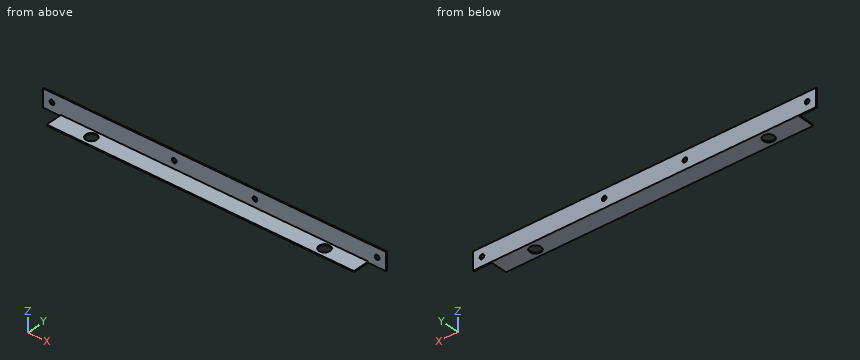
```python
from build123d import *

# Parameters (mm, degrees)
F1_DEPTH = 242.8875
F2_R     = 7.9375
F2_W     = 25.4
F2_H     = 23.8125
F4_DEPTH = 25.4
F3_R     = 3.302
F5_DEPTH = 25.4


with BuildPart() as f1:
    # F0 (on Right) → F1 (new body, symmetric)
    with BuildSketch(Plane.YZ):
        Polygon((0, 0), (0, 25.4), (-1.5875, 25.4), (-1.5875, 1.5875), (-25.4, 1.5875), (-25.4, 0), align=None)
    extrude(amount=F1_DEPTH, both=True)

    # F2 (on face) → F4 (cut)
    with BuildSketch(Plane(origin=(0, 0, 0), x_dir=(1, 0, 0), z_dir=(0, 0, -1))):
        with Locations((-165.1, 12.7)):
            Circle(F2_R)
        with Locations((165.1, 12.7)):
            Circle(F2_R)
        with Locations((-230.1875, 13.49375)):
            Rectangle(F2_W, F2_H)
        with Locations((230.1875, 13.49375)):
            Rectangle(F2_W, F2_H)
    extrude(amount=-F4_DEPTH, mode=Mode.SUBTRACT)

    # F3 (on face) → F5 (cut)
    with BuildSketch(Plane.XZ.offset(1.5875)):
        with Locations((-230.1875, 12.7)):
            Circle(F3_R)
        with Locations((230.1875, 12.7)):
            Circle(F3_R)
        with Locations((-57.15, 12.7)):
            Circle(F3_R)
        with Locations((57.15, 12.7)):
            Circle(F3_R)
    extrude(amount=-F5_DEPTH, mode=Mode.SUBTRACT)


solid = f1.part
```
Part model, mm, in its own coordinate system. Coordinates: 2 decimals unless noted, no trailing zeros. Order: outer loops, then holes, each group sorted by start corner. A loop starts at its lowest first (then second) coordinate and runs counter-clockwise, first axis right, second up. Notation, with made-up numbers: (64, 63) - (79, 63) arc R10 ccw to (79, 80) - close; hole circle Ø8 at (33, -18). An arc over 180 degrees is marked (long way). Return JSON: item names as keys, results as strings. Group by question number.
Item 1: Cut at B-B (x = -165.1). List the corners of the cut face in (y, z).
Item 2: Pin check, flat tips, straight feed: pin 1 (6 mm diameter, centred on x = -170.5, y = -10.5, fed in from +Z); pin 2 (6 mm diameter, centred on x = -57.15, z = 12.7, fed in from +Y) (1 decimal); pin 3 (7.5 mm diameter, centred on x = 57.15, z = 12.7, fed in from -Y); pin 4 (0.8 mm diameter, centred on y = -10.5, z = 1, fed in from +X). Stop position of each tip, or through.
Item 3: Cut at C-C (x = 211). List the corners of the cut face in (y, z), plus the area to 3 significant figures.
Item 4: Cut at A-A (y = -12.7). List the corners of the cut face in (x, z), plus the area to 3 significant figures.
Item 5: Drill centre lines: probe 1 along X at (y, z) = (-12.7, 1.05); probe 2 along Y at (x, z) = (-165.1, 1.2); probe 3 along Y at (x, z) = (-17, 12.25). Where is each one in solid material? Low to high. Write a range as from..to.
Check values:
{
 "1": {"outline": "(-25.4, 0) - (-20.64, 0) - (-20.64, 1.59) - (-25.4, 1.59) - close; (-4.76, 0) - (0, 0) - (0, 25.4) - (-1.59, 25.4) - (-1.59, 1.59) - (-4.76, 1.59) - close"},
 "2": {"pin 1": "stops at z = 1.59", "pin 2": "passes through", "pin 3": "stops at y = -1.59", "pin 4": "stops at x = 217.49"},
 "3": {"outline": "(-25.4, 0) - (0, 0) - (0, 25.4) - (-1.59, 25.4) - (-1.59, 1.59) - (-25.4, 1.59) - close", "area": "78.1 mm2"},
 "4": {"outline": "(-217.49, 0) - (-173.04, 0) - (-173.04, 1.59) - (-217.49, 1.59) - close; (-157.16, 0) - (157.16, 0) - (157.16, 1.59) - (-157.16, 1.59) - close; (173.04, 0) - (217.49, 0) - (217.49, 1.59) - (173.04, 1.59) - close", "area": "640 mm2"},
 "5": {"probe 1": "x = -217.49..-173.04, -157.16..157.16, 173.04..217.49", "probe 2": "y = -25.4..-20.64, -4.76..0", "probe 3": "y = -1.59..0"}
}
